Could you check a few things on this drawing? It's one solid part, dimensions in mm from its lowest x, y, z. A direction names the side the tool comes from. Round coordinates to 2 decimals unless told otherwise and drop trailing zeros. Loops run counter-clockwise (first coordinate to the right, second up) from the corner with the lowest first, then second, coordinate; pieces in that order, holes last. Notation, with made-up numbers: (38.5, -11.75) -> (47.5, -11.75) arc R31 cw to (47.5, 19.25) -> close; hole circle Ø7 at (-26, 87). An arc over 180 degrees is marked (long way). Use one line per item in the form item = value. Start each with the question number.
Item 1: If we section it at A-A (y = 3.25): Write out the boundary of the cut face in (x, z).
Item 2: If I drill on L1, parallel to Y at x = 2.5, z = 3.8; L2, parallel to Z at x = 2.5, y = 2.65; L3, parallel to Y at x = 2, z = 1.5, over which ranges is the centre line in solid material (lowest first)? Write a range as [from, to].
Item 3: For the marked faces 4, 5 and 6, which set-ups out of +Z, -Z, +X, -X, +Y, -Y let a thin tool reach every point of the face, with its end or its side?
Item 4: I'm going to push a flat-ended pin straight in: pin 1 Ø0.6 at (x, y) = (5.5, 2.5) entering from +Z. Where does the tip first touch, or does it pass through?
Item 5: Thinking about a two-plate mould opening in X: for the marked faces 1, 2 and 3, which applies, released by +X, released by -X, zero draft, split by the parting line, or undercut?
Item 6: If we section it at C-C (z = 1.85): Write out the boundary of the cut face in (x, y).
Item 7: If we section it at D-D (y = 1.5): Write out the boundary of the cut face in (x, z), then the cut area to 3 significant figures.
Item 8: If we section it at B-B (x = 3.5): Write out the boundary of the cut face in (y, z), then the cut area to 3 significant figures.
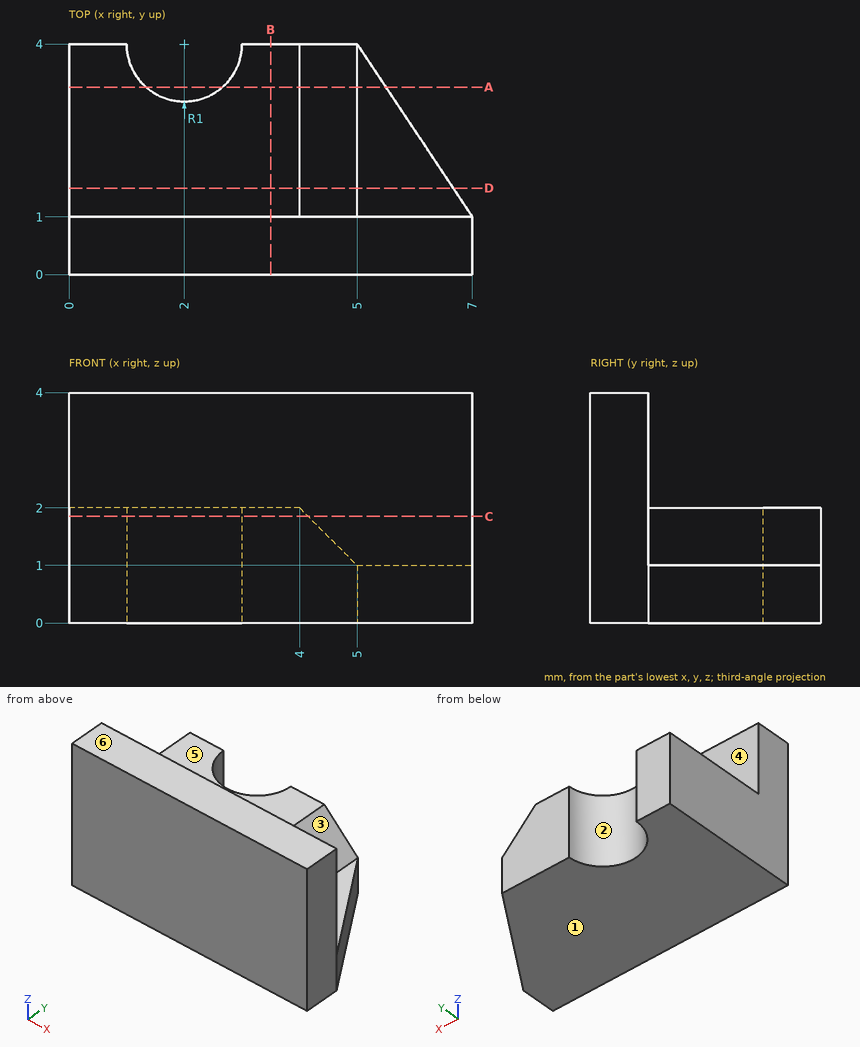
Values found:
q1.outline = (0, 0) -> (1.34, 0) -> (1.34, 2) -> (0, 2) -> close; (2.66, 0) -> (5.5, 0) -> (5.5, 1) -> (5, 1) -> (4, 2) -> (2.66, 2) -> close
q2.L1 = [0, 1]
q2.L2 = [0, 2]
q2.L3 = [0, 3]
q3.face_4 = +Z, +X, +Y
q3.face_5 = +Z, +X, -X, +Y
q3.face_6 = +Z, +X, -X, +Y, -Y
q4.pin_1 = 1
q5.face_1 = zero draft
q5.face_2 = undercut
q5.face_3 = released by +X
q6.outline = (0, 0) -> (7, 0) -> (7, 1) -> (4.15, 1) -> (4.15, 4) -> (3, 4) arc R1 cw to (1, 4) -> (0, 4) -> close
q7.outline = (0, 0) -> (6.67, 0) -> (6.67, 1) -> (5, 1) -> (4, 2) -> (0, 2) -> close
q7.area = 11.2 mm2
q8.outline = (0, 0) -> (4, 0) -> (4, 2) -> (1, 2) -> (1, 4) -> (0, 4) -> close
q8.area = 10.0 mm2
